Answer from the drawing. Dimensions are ordinates in mm from the lowest x, y and z of the part. A direction names the side the tool comes from. Coordinates: 2 decimals unless noted, no trailing zeros. Loops run counter-clockwise (first coordinate to the right, second up) from the corner with the lowest first, then second, coordinate; pieces in that order, holes last.
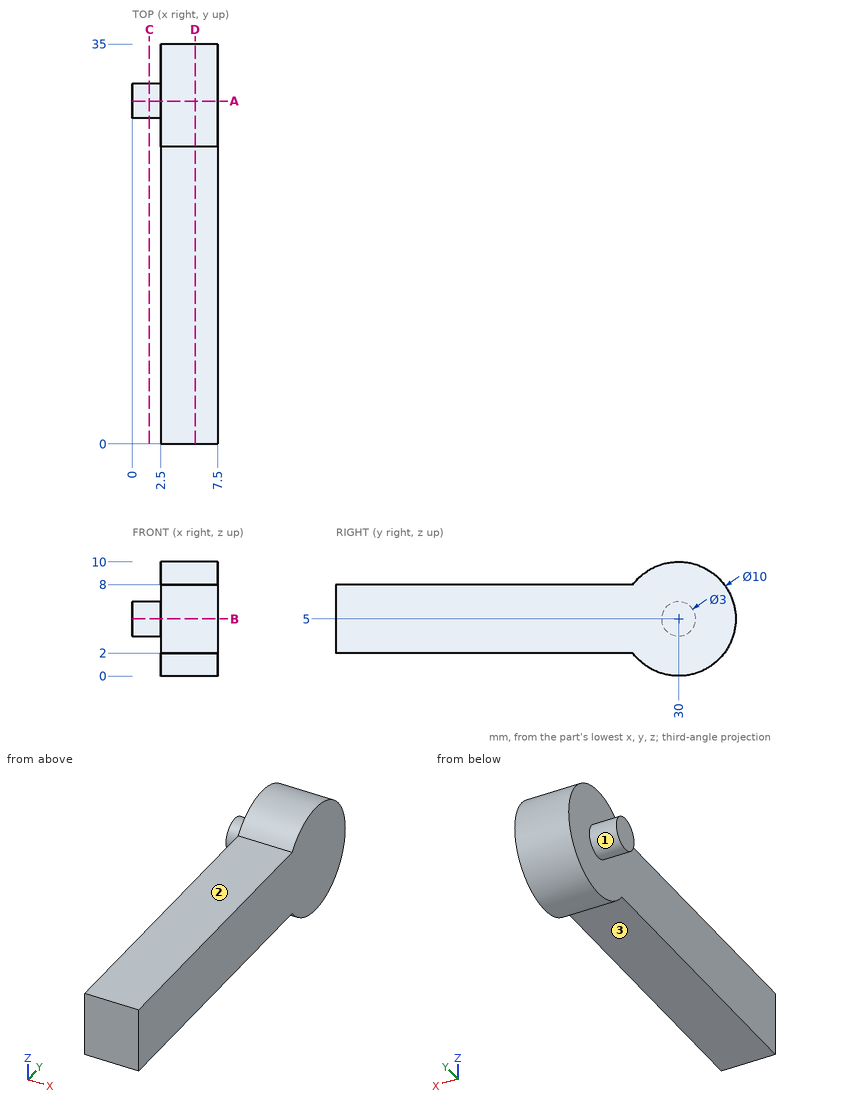
Item 1: A cutting plane is placed at C-C on x = 1.5. Determine the outline of the cut face in (y, z).
Numbers:
outline: circle Ø3 at (30, 5)
Item 2: A cutting plane is placed at B-B on z = 5. Determine the outline of the cut face in (x, y).
Numbers:
outline: (0, 28.5) - (2.5, 28.5) - (2.5, 0) - (7.5, 0) - (7.5, 35) - (2.5, 35) - (2.5, 31.5) - (0, 31.5) - close
Item 3: A cutting plane is placed at D-D on x = 5.5. Determine the outline of the cut face in (y, z), then the cut area to 3 significant figures.
Numbers:
outline: (0, 2) - (26, 2) arc R5 ccw (long way) to (26, 8) - (0, 8) - close
area: 230 mm2
Item 4: A cutting plane is placed at A-A on y = 30. Determine the outline of the cut face in (x, z), then the cut area to 3 significant figures.
Numbers:
outline: (0, 3.5) - (2.5, 3.5) - (2.5, 0) - (7.5, 0) - (7.5, 10) - (2.5, 10) - (2.5, 6.5) - (0, 6.5) - close
area: 57.5 mm2
Item 5: Find the intervals of material crossed by line 1 along X through (y, z) = (11.5, 4.25); line 2 along Z through (x, y) = (4.25, 10.5); line 3 along Y through (x, z) = (3, 1.25), in increasing order.
Numbers:
line 1: x = 2.5 to 7.5
line 2: z = 2 to 8
line 3: y = 26.69 to 33.31
Item 6: Which of the six approach directions +Z, -Z, +X, -X, +Y, -Y give full straight-line access (tool end or side, diameter ignored) to the marked faces 1, 2 and 3?
Numbers:
face 1: -X
face 2: +Z, +X, -X, -Y
face 3: -Z, +X, -X, -Y
Item 7: Given pin 1 (6 mm diameter, centred on y = 24, z = 1, fed in from +X); pin 2 (2 mm diameter, centred on y = 11, z = 6, fed in from -X); pin 3 (2.5 mm diameter, centred on x = 5.5, y = 15.5, fed in from +Z); pin 4 (1.5 mm diameter, centred on x = 5, y = 13.5, fed in from -Z), each flat-ended and moving along its own axis, determine where each tip first touches the part or whether it passes through.
Numbers:
pin 1: stops at x = 7.5
pin 2: stops at x = 2.5
pin 3: stops at z = 8
pin 4: stops at z = 2
